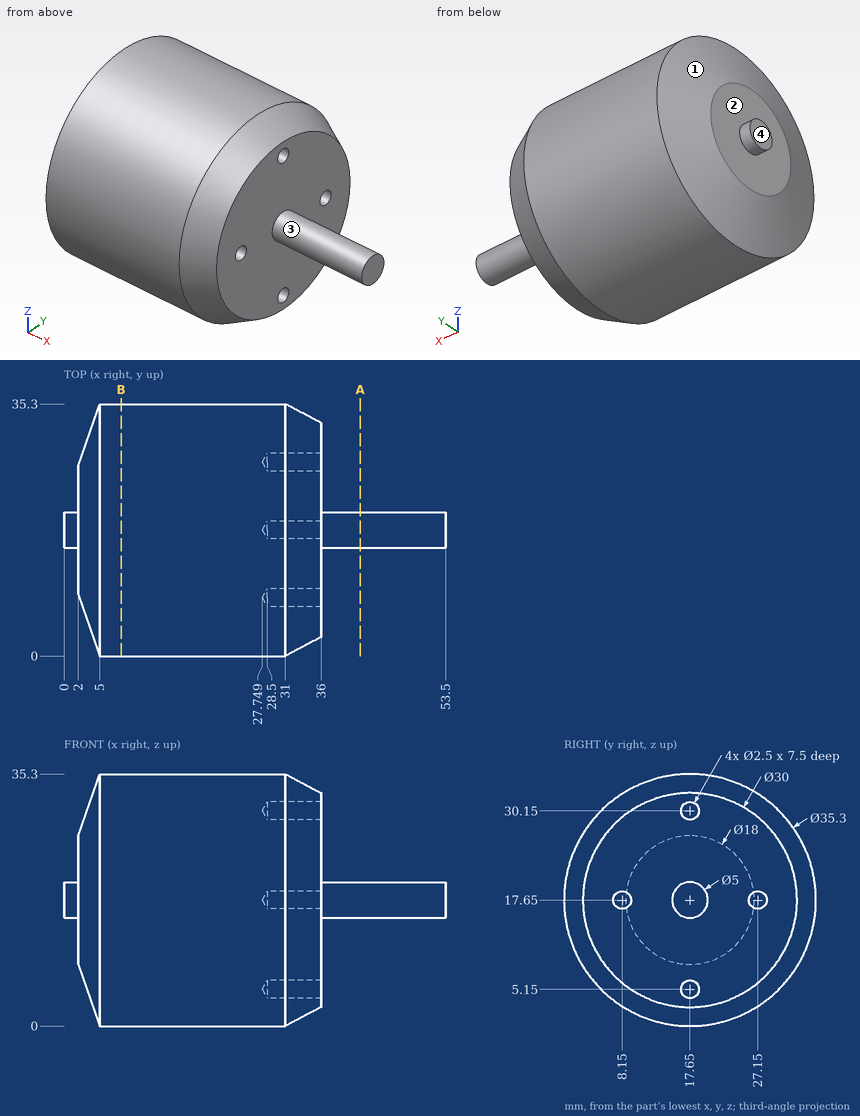
Geometry check sheet. Reference: drawing and pictorial views, mm from the part's lowest x, y, z. A direction names the side the tool comes from. Round coordinates to 2 decimals unless told otherwise and drop trailing zeros. Loops run counter-clockwise (first coordinate to the right, second up) from the corner with the lowest first, then second, coordinate; pieces in that order, holes last. Notation, with made-up numbers: (64.25, 87.25) - (96.25, 87.25) arc R12 ccw to (96.25, 91.25) - close; hole circle Ø8 at (20, 77). An arc over 180 degrees is marked (long way). Use a Markdown table: item, result.
Q1. Draft check along Y on the marked faces 1 and 2. Enter one of: released by +Y, released by -Y, zero draft, split by the parting line, or undercut.
Solutions:
| item | result |
|---|---|
| face 1 | split by the parting line |
| face 2 | zero draft |
Q2. Cross-section at B-B on x = 8. Record the cut outline in (y, z), plus the area to 3 significant figures.
Solutions:
| item | result |
|---|---|
| outline | circle Ø35.3 at (17.65, 17.65) |
| area | 979 mm2 |
Q3. Access from +Z, -Z, +X, -X, +Y, -Y to the whole of each face (thin tool, end or side, straight path). Record for the marked faces 3 and 4.
Solutions:
| item | result |
|---|---|
| face 3 | +X |
| face 4 | +Z, -Z, -X, +Y, -Y |
Q4. Material ranges on line 1 (Y direction, x = 31.25, z = 17.65); line 2 (Z direction, x = 33, y = 17); line 3 (Z direction, x = 30, y = 17), recorded low to high.
Solutions:
| item | result |
|---|---|
| line 1 | y = 0.13 to 6.9, 9.4 to 25.9, 28.4 to 35.17 |
| line 2 | z = 1.07 to 4.08, 6.22 to 29.08, 31.22 to 34.23 |
| line 3 | z = 0.01 to 4.08, 6.22 to 29.08, 31.22 to 35.29 |
Q5. Go/stop test with flat-tipped pins: P1, Ø4, axis at x = 33.5, z = 15.5, coming from the +Y side; P2, Ø3, axis at y = 17.65, z = 5.15, coming from the -X side; P3, Ø2, axis at y = 8.15, z = 17.65, coming from the -X side. Record where each tip stops, or that it passes through.
Solutions:
| item | result |
|---|---|
| P1 | stops at y = 34.93 |
| P2 | stops at x = 2.69 |
| P3 | stops at x = 2 |
Q6. Cross-section at A-A on x = 41.5. Record the cut outline in (y, z).
Solutions:
| item | result |
|---|---|
| outline | circle Ø5 at (17.65, 17.65) |
